Work out the finished part from the listing and answer in its coordinate system (mm). Face numbers are marked on the shaded views. Give positions to 0.01 mm unless a question says otherwise; leave off trailing zeros. Loops run counter-clockwise (first coordinate to the right, second up) from the corner with the lowest first, then second, coordinate; pieces in that order, holes last. Notation, with made-up numbers: M 31.5,66 L 46.5,66 A10 ccw 46.5,77 Z; hole C -14,-20.75 d7. An arc over 180 degrees is marked long. Use a Markdown table: item, result.
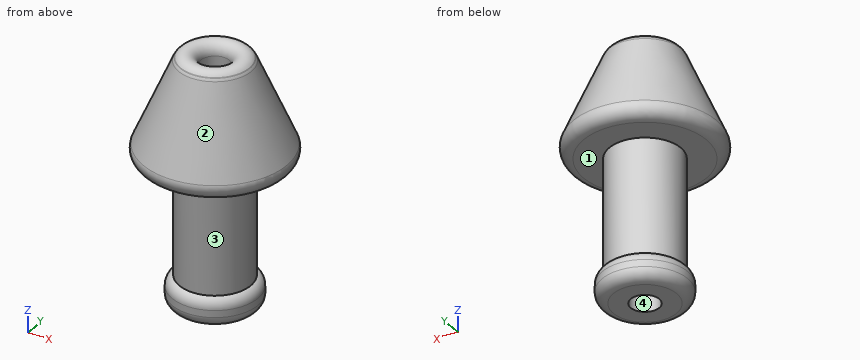
```python
from build123d import *

# Parameters (mm, degrees)
F0_W = 0.5
F0_H = 2


# Not quite as in the source:
# - a fillet or chamfer that OpenCascade refuses, or shapes differently, is made with other operations: its cross-section is extruded or revolved along the edge and cut away or added


with BuildPart() as f1:
    # F0 (on Front) → F1 (revolve)
    with BuildSketch(Plane.XZ):
        Polygon((-2.5, 0), (-1, 0), (-1, 18.7049116939), (-2.5, 16.9229302555), (-5.5, 10), (-2.5, 10), (-2.5, 2), align=None)
        with Locations((-2.75, 1)):
            Rectangle(F0_W, F0_H)
    revolve(axis=Axis((0, 0, 13.3904740214), (0, 0, 1)))

    # F2: fillet of radius 0.8 on 5 edges, made by hand

    # F2_s1 → F2_t2 (revolve, cut)
    with BuildSketch(Plane.XZ):
        with BuildLine():
            ThreePointArc((-2.424695214, 17.0126243355), (-2.4928760132, 16.918520212), (-2.546704077, 16.8155311495))
            Line((-2.546704077, 16.8155311495), (-2.5613849178, 16.821892982))
            ThreePointArc((-2.5613849178, 16.821892982), (-2.5379640629, 16.8755627139), (-2.5146808408, 16.929292088))
            Line((-2.5146808408, 16.929292088), (-2.5122406636, 16.9332339517))
            ThreePointArc((-2.5122406636, 16.9332339517), (-2.4745308925, 16.9780326932), (-2.4369358776, 17.0229280317))
            Line((-2.4369358776, 17.0229280317), (-2.424695214, 17.0126243355))
        make_face()
    revolve(axis=Axis((0, 0, 16.9229302555), (0, 0, 1)), mode=Mode.SUBTRACT)

    # F2_s3 → F2_t4 (revolve, cut)
    with BuildSketch(Plane.XZ):
        with BuildLine():
            ThreePointArc((-5.0157118449, 11.1179416236), (-4.9504273448, 10.3608017674), (-4.2816698032, 9.99985))
            Line((-4.2816698032, 9.99985), (-4.2816698032, 9.98385))
            ThreePointArc((-4.2816698032, 9.98385), (-4.8908349016, 9.984), (-5.5, 9.984))
            Line((-5.5, 9.984), (-5.5146808408, 10.0063618325))
            ThreePointArc((-5.5146808408, 10.0063618325), (-5.2724679468, 10.5653028232), (-5.0303926857, 11.1243034561))
            Line((-5.0303926857, 11.1243034561), (-5.0157118449, 11.1179416236))
        make_face()
    revolve(axis=Axis((0, 0, 10), (0, 0, 1)), mode=Mode.SUBTRACT)

    # F2_s5 → F2_t6 (revolve, cut)
    with BuildSketch(Plane.XZ):
        with BuildLine():
            ThreePointArc((-0.99985, 16.5126600652), (-1.5256480152, 17.2642006639), (-2.4118831788, 17.0278448749))
            Line((-2.4118831788, 17.0278448749), (-2.4241238423, 17.0381485711))
            ThreePointArc((-2.4241238423, 17.0381485711), (-1.7181248748, 17.876633682), (-1.0122406636, 18.7152153901))
            Line((-1.0122406636, 18.7152153901), (-0.984, 18.7049116939))
            ThreePointArc((-0.984, 18.7049116939), (-0.984, 17.6087858796), (-0.98385, 16.5126600652))
            Line((-0.98385, 16.5126600652), (-0.99985, 16.5126600652))
        make_face()
    revolve(axis=Axis((0, 0, 18.7049116939), (0, 0, 1)), mode=Mode.SUBTRACT)

    # F2_s7 → F2_t8 (revolve, cut)
    with BuildSketch(Plane.XZ):
        with BuildLine():
            ThreePointArc((-2.5000562324, 2.0001390608), (-2.8634466855, 1.7057368158), (-3.00015, 1.2584812882))
            Line((-3.00015, 1.2584812882), (-3.01615, 1.2584812882))
            ThreePointArc((-3.01615, 1.2584812882), (-3.016, 1.6292406441), (-3.016, 2))
            Line((-3.016, 2), (-3, 2.016))
            ThreePointArc((-3, 2.016), (-2.7500281162, 2.016), (-2.5060543571, 2.0149722163))
            Line((-2.5060543571, 2.0149722163), (-2.5000562324, 2.0001390608))
        make_face()
    revolve(axis=Axis((0, 0, 2), (0, 0, 1)), mode=Mode.SUBTRACT)

    # F2_s9 → F2_t10 (revolve, cut)
    with BuildSketch(Plane.XZ):
        with BuildLine():
            ThreePointArc((-3.00015, 0.79985), (-2.7658354249, 0.2341645751), (-2.20015, -0.00015))
            Line((-2.20015, -0.00015), (-2.20015, -0.01615))
            ThreePointArc((-2.20015, -0.01615), (-2.600075, -0.016), (-3, -0.016))
            Line((-3, -0.016), (-3.016, 0))
            ThreePointArc((-3.016, 0), (-3.016, 0.399925), (-3.01615, 0.79985))
            Line((-3.01615, 0.79985), (-3.00015, 0.79985))
        make_face()
    revolve(axis=Axis((0, 0, 0), (0, 0, 1)), mode=Mode.SUBTRACT)


solid = f1.part
```
(1) Consider probe 1 along X at (y, z) = (0, 5.5); probe 2 along Y at (x, z) = (0, 10.5). Determine where each line is inside the solid, lowest interval first. Write a range as [from, to].
Entries:
| item | result |
|---|---|
| probe 1 | x = [-2.5, -1], [1, 2.5] |
| probe 2 | y = [-5.02, -1], [1, 5.02] |
(2) The mould has two halves that part along Z. Classify the marked faces 1, 2, 3 and 4: released by +Z, released by -Z, zero draft, split by the parting line, or undercut.
Entries:
| item | result |
|---|---|
| face 1 | undercut |
| face 2 | released by +Z |
| face 3 | undercut |
| face 4 | zero draft |
(3) Given P1, Ø1, axis at x = 2, z = 12, coming from the +Y side; P2, Ø2, axis at x = -2, y = -2, coming from the -Z side; P3, Ø3, axis at x = 0, y = 0, coming from the +Z side; P4, Ø3, axis at y = -2, z = 3, coming from the -X side, each flat-ended and moving along its own axis, determine where each tip first touches the part or whether it passes through.
Entries:
| item | result |
|---|---|
| P1 | stops at y = 4.5 |
| P2 | stops at z = 0 |
| P3 | stops at z = 17.25 |
| P4 | stops at x = -2.58 |
(4) A cutting plane is placed at B-B (z = 5.75). Write down the section's boundary in (x, y), and give its area (3 significant figures).
Entries:
| item | result |
|---|---|
| outline | C 0,0 d5; hole C 0,0 d2 |
| area | 16.5 mm² |
(5) A cutting plane is placed at C-C (z = 10.25). Write down the section's boundary in (x, y), and give its area (3 significant figures).
Entries:
| item | result |
|---|---|
| outline | C 0,0 d9.73; hole C 0,0 d2 |
| area | 71.1 mm² |
